Model file for the job. Use its own axes, mm. Face numbers are marked on the shaded views. A direction names the side the tool comes from. Coordinates: 2 decimals unless noted, no trailing zeros. Write each loop counter-clockwise with the first axis right and the second up, starting at its lowest first coordinate (ties: lowest second). Pieces come first, ordered by that corner, then holes. Notation, with made-up numbers: (65, 59.25) - (76, 59.25) arc R23 ccw to (76, 90.25) - close; hole circle Ø6 at (61.5, 86.25). An arc over 180 degrees is marked (long way). Put each result on its own line as item: value. Start each with the question number.
1. Which spindle directions (+Z, -Z, +X, -X, +Y, -Y) get a long thin tool onto all of the face, cutting with end or side? Do the marked faces 4, 5 and 6. Say none if no direction does.
2. Saw through at B-B, the plane y = 3.25. Write the cut outline in (x, z).
3. Saw through at A-A, the plane y = 0. Write the cut outline in (x, z).
4. Saw through at D-D, the plane x = 3. Write the cut outline in (y, z), plus the area to 3 significant figures.
5. Drop flat-ended pins along their axis: P1, Ø3, axis at y = 7.5, z = 3.5, coming from the -X side; P2, Ø3.5, axis at x = 3, y = 7.5, coming from the +Z side; P3, Ø4, axis at x = 1.5, y = 3, coming from the +Z side. Give the stop position or say it passes through.
6. Drill centre lines: L1, parallel to Z at x = -5.25, y = 6; L2, parallel to X at y = 11.75, z = 8.25; L3, parallel to Y at x = 0, z = 0.35. Where is each one in solid material? Low to high. Write a range as from..to.
7. Saw through at C-C, the plane z = 3.75. Write the cut outline in (x, y), plus the area to 3 significant figures.
8. Pull direction X, two halves, no side cores. Call the marked faces 1, 2 and 3: released by +X, released by -X, zero draft, split by the parting line, or undercut.
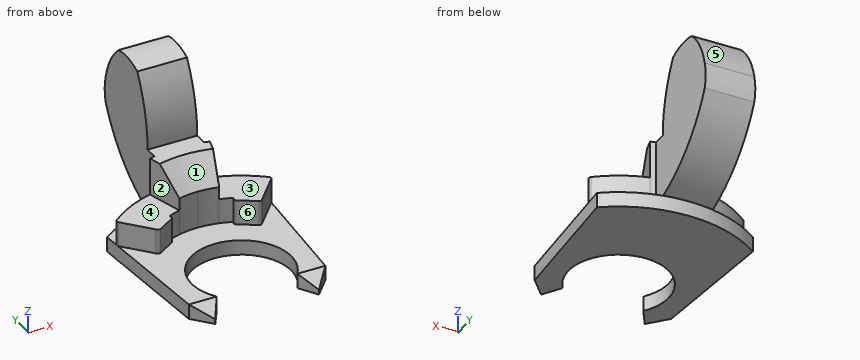
```python
from build123d import *

# Parameters (mm, degrees)
F1_DEPTH    = 1.2
F3_DEPTH    = 12.5
F5_DEPTH    = 2
F6_DEPTH    = 5
F7_T2_ANGLE = 119.2786087223
F8_DEPTH    = 5
F10_DEPTH   = 4
F11_DEPTH   = 5


# Not quite as in the source:
# - a fillet or chamfer that OpenCascade refuses, or shapes differently, is made with other operations: its cross-section is extruded or revolved along the edge and cut away or added
# - a feature names something its author has since deleted; it is built from what else it names


with BuildPart() as f1:
    # F0 (on Top) → F1 (new body)
    with BuildSketch(Plane.XY):
        with BuildLine():
            ThreePointArc((-3.25, -2.3318447633), (0, 4), (3.25, -2.3318447633))
            Line((3.25, -2.3318447633), (4.1771243445, -3.8318447633))
            Line((4.1771243445, -3.8318447633), (5.5, -2.3318447633))
            Line((5.5, -2.3318447633), (6.2861850371, 8.4103434936))
            ThreePointArc((6.2861850371, 8.4103434936), (0, 10.5), (-6.2861850371, 8.4103434936))
            Line((-6.2861850371, 8.4103434936), (-5.5, -2.3318447633))
            Line((-5.5, -2.3318447633), (-4.1771243445, -3.8318447633))
            Line((-4.1771243445, -3.8318447633), (-3.25, -2.3318447633))
        make_face()
    extrude(amount=F1_DEPTH)

    # F2 (on Right) → F3 (cut, symmetric)
    with BuildSketch(Plane.YZ):
        Polygon((-3.8318447633, 0.4), (-2.3318447633, 1.2), (-3.8318447633, 1.2), align=None)
    extrude(amount=F3_DEPTH, both=True, mode=Mode.SUBTRACT)

    # F4 (on face) → F5 (join)
    with BuildSketch(Plane.XY.offset(1.2)):
        with BuildLine():
            Line((0, 9.4893432962), (0, 9.5))
            ThreePointArc((0, 9.5), (-1.0056504861, 9.4466219941), (-2, 9.2870878105))
            ThreePointArc((-2, 9.2870878105), (-2.207287093, 9.2400153511), (-2.4134691055, 9.1883168686))
            Line((-2.4134691055, 9.1883168686), (-1.6054997382, 6.2986006851))
            ThreePointArc((-1.6054997382, 6.2986006851), (-0.809041268, 6.4494536378), (0, 6.5))
            Line((0, 6.5), (0, 9.4893432962))
        make_face()
        with BuildLine():
            Line((0, 10.3126084432), (0, 9.5))
            ThreePointArc((0, 9.5), (1.0056504861, 9.4466219941), (2, 9.2870878105))
            Line((2, 9.2870878105), (2, 10.3126084432))
            Line((2, 10.3126084432), (0, 10.3126084432))
        make_face()
        with BuildLine():
            ThreePointArc((2, 9.2870878105), (1.0056504861, 9.4466219941), (0, 9.5))
            Line((0, 9.5), (0, 9.4893432962))
            Line((0, 9.4893432962), (0, 6.5))
            ThreePointArc((0, 6.5), (0.809041268, 6.4494536378), (1.6054997382, 6.2986006851))
            Line((1.6054997382, 6.2986006851), (2.4134691055, 9.1883168686))
            ThreePointArc((2.4134691055, 9.1883168686), (2.207287093, 9.2400153511), (2, 9.2870878105))
        make_face()
        with BuildLine():
            ThreePointArc((-2, 9.2870878105), (-1.0056504861, 9.4466219941), (0, 9.5))
            Line((0, 9.5), (0, 10.3126084432))
            Line((0, 10.3126084432), (-2, 10.3126084432))
            Line((-2, 10.3126084432), (-2, 9.2870878105))
        make_face()
        with BuildLine():
            Line((-1.6054997382, 6.2986006851), (-2.4134691055, 9.1883168686))
            ThreePointArc((-2.4134691055, 9.1883168686), (-4.3834961594, 8.4282240965), (-6.1369591907, 7.2517399217))
            ThreePointArc((-6.1369591907, 7.2517399217), (-6.2072372931, 7.1135226449), (-6.1576144754, 6.9666192642))
            Line((-6.1576144754, 6.9666192642), (-4.3047045796, 4.8702688306))
            Line((-4.3047045796, 4.8702688306), (-4.2185888433, 4.7728389657))
            ThreePointArc((-4.2185888433, 4.7728389657), (-4.0971505607, 4.7073203992), (-3.9621862374, 4.7360357341))
            Line((-3.9621862374, 4.7360357341), (-2.5827247856, 5.6044208159))
            ThreePointArc((-2.5827247856, 5.6044208159), (-2.4942501859, 5.7293355978), (-2.5200172859, 5.8802246764))
            Line((-2.5200172859, 5.8802246764), (-2.5753119947, 5.968062343))
            ThreePointArc((-2.5753119947, 5.968062343), (-2.096928846, 6.152470188), (-1.6054997382, 6.2986006851))
        make_face()
        with BuildLine():
            ThreePointArc((6.1369591907, 7.2517399217), (4.3834961594, 8.4282240965), (2.4134691055, 9.1883168686))
            Line((2.4134691055, 9.1883168686), (1.6054997382, 6.2986006851))
            ThreePointArc((1.6054997382, 6.2986006851), (2.096928846, 6.152470188), (2.5753119947, 5.968062343))
            Line((2.5753119947, 5.968062343), (2.5200172859, 5.8802246764))
            ThreePointArc((2.5200172859, 5.8802246764), (2.4942501859, 5.7293355978), (2.5827247856, 5.6044208159))
            Line((2.5827247856, 5.6044208159), (3.9621862374, 4.7360357341))
            ThreePointArc((3.9621862374, 4.7360357341), (4.0971505607, 4.7073203992), (4.2185888433, 4.7728389657))
            Line((4.2185888433, 4.7728389657), (4.3047045796, 4.8702688306))
            Line((4.3047045796, 4.8702688306), (6.1576144754, 6.9666192642))
            ThreePointArc((6.1576144754, 6.9666192642), (6.2072372931, 7.1135226449), (6.1369591907, 7.2517399217))
        make_face()
    extrude(amount=F5_DEPTH)

    # F4 (on face) → F6 (join)
    with BuildSketch(Plane.XY.offset(1.2)):
        with BuildLine():
            ThreePointArc((2, 9.2870878105), (1.0056504861, 9.4466219941), (0, 9.5))
            Line((0, 9.5), (0, 9.4893432962))
            Line((0, 9.4893432962), (0, 6.5))
            ThreePointArc((0, 6.5), (0.809041268, 6.4494536378), (1.6054997382, 6.2986006851))
            Line((1.6054997382, 6.2986006851), (2.4134691055, 9.1883168686))
            ThreePointArc((2.4134691055, 9.1883168686), (2.207287093, 9.2400153511), (2, 9.2870878105))
        make_face()
        with BuildLine():
            Line((0, 9.4893432962), (0, 9.5))
            ThreePointArc((0, 9.5), (-1.0056504861, 9.4466219941), (-2, 9.2870878105))
            ThreePointArc((-2, 9.2870878105), (-2.207287093, 9.2400153511), (-2.4134691055, 9.1883168686))
            Line((-2.4134691055, 9.1883168686), (-1.6054997382, 6.2986006851))
            ThreePointArc((-1.6054997382, 6.2986006851), (-0.809041268, 6.4494536378), (0, 6.5))
            Line((0, 6.5), (0, 9.4893432962))
        make_face()
    extrude(amount=F6_DEPTH)

    # F7: chamfer of 2 on 1 edges, made by hand

    # F7_s1 → F7_t2 (revolve, cut)
    with BuildSketch(Plane(origin=(0, 0, 0), x_dir=(0, 0, 1), z_dir=(-0.5054419689, -0.8628606006, 0))):
        Polygon((6.2, 8.5), (4.2, 6.5), (6.2, 6.5), align=None)
    revolve(axis=Axis((0, 0, 6.2), (0, 0, -1)), revolution_arc=F7_T2_ANGLE, mode=Mode.SUBTRACT)

    # F4 (on face) → F8 (join, through all)
    with BuildSketch(Plane.XY.offset(1.2)):
        with BuildLine():
            Line((0, 10.3126084432), (0, 9.5))
            ThreePointArc((0, 9.5), (1.0056504861, 9.4466219941), (2, 9.2870878105))
            Line((2, 9.2870878105), (2, 10.307764064))
            ThreePointArc((2, 10.307764064), (1.9874359165, 10.3101939108), (1.974868881, 10.3126084432))
            Line((1.974868881, 10.3126084432), (0, 10.3126084432))
        make_face()
        with BuildLine():
            ThreePointArc((1.974868881, 10.3126084432), (1.9874359165, 10.3101939108), (2, 10.307764064))
            Line((2, 10.307764064), (2, 10.3126084432))
            Line((2, 10.3126084432), (1.974868881, 10.3126084432))
        make_face()
        with BuildLine():
            Line((-2, 10.3126084432), (-2, 10.307764064))
            ThreePointArc((-2, 10.307764064), (-1.9874359165, 10.3101939108), (-1.974868881, 10.3126084432))
            Line((-1.974868881, 10.3126084432), (-2, 10.3126084432))
        make_face()
        with BuildLine():
            ThreePointArc((-2, 9.2870878105), (-1.0056504861, 9.4466219941), (0, 9.5))
            Line((0, 9.5), (0, 10.3126084432))
            Line((0, 10.3126084432), (-1.974868881, 10.3126084432))
            ThreePointArc((-1.974868881, 10.3126084432), (-1.9874359165, 10.3101939108), (-2, 10.307764064))
            Line((-2, 10.307764064), (-2, 9.2870878105))
        make_face()
    extrude(amount=F8_DEPTH)

    # F9 (on face) → F10 (join)
    with BuildSketch(Plane(origin=(-2, 0, 0), x_dir=(0, -1, 0), z_dir=(-1, 0, 0))):
        with BuildLine():
            Line((-10.4906475171, 1.2), (-10.3126084432, 1.2))
            Line((-10.3126084432, 1.2), (-10.3126084432, 6.2))
            ThreePointArc((-10.3126084432, 6.2), (-10.7033019047, 9.142871965), (-11.848315427, 11.8818646297))
            ThreePointArc((-11.848315427, 11.8818646297), (-13.2228522743, 12.2616673302), (-14.6442650052, 12.1468305588))
            ThreePointArc((-14.6442650052, 12.1468305588), (-15.8696799602, 10.6519801079), (-16.5821556002, 8.8551500812))
            ThreePointArc((-16.5821556002, 8.8551500812), (-16.7217466821, 7.8095628414), (-16.5821556002, 6.7639756016))
            ThreePointArc((-16.5821556002, 6.7639756016), (-14.0870903715, 3.3790869985), (-10.4906475171, 1.2))
        make_face()
    extrude(amount=-F10_DEPTH)

    # F4 (on face) → F11 (join, through all)
    with BuildSketch(Plane.XY.offset(1.2)):
        with BuildLine():
            Line((0, 10.3126084432), (0, 9.5))
            ThreePointArc((0, 9.5), (1.0056504861, 9.4466219941), (2, 9.2870878105))
            Line((2, 9.2870878105), (2, 10.307764064))
            ThreePointArc((2, 10.307764064), (1.9874359165, 10.3101939108), (1.974868881, 10.3126084432))
            Line((1.974868881, 10.3126084432), (0, 10.3126084432))
        make_face()
        with BuildLine():
            ThreePointArc((-2, 9.2870878105), (-1.0056504861, 9.4466219941), (0, 9.5))
            Line((0, 9.5), (0, 10.3126084432))
            Line((0, 10.3126084432), (-1.974868881, 10.3126084432))
            ThreePointArc((-1.974868881, 10.3126084432), (-1.9874359165, 10.3101939108), (-2, 10.307764064))
            Line((-2, 10.307764064), (-2, 9.2870878105))
        make_face()
    extrude(amount=F11_DEPTH)


solid = f1.part
```
Final values:
1. face 4: +Z, -X, -Y
1. face 5: +Z, +X, -X, +Y
1. face 6: +Z, -Y
2. outline: (-5.91, 0) - (-2.33, 0) - (-2.33, 1.2) - (-5.91, 1.2) - close; (2.33, 0) - (5.91, 0) - (5.91, 1.2) - (2.33, 1.2) - close
3. outline: (-5.67, 0) - (-4, 0) - (-4, 1.2) - (-5.67, 1.2) - close; (4, 0) - (5.67, 0) - (5.67, 1.2) - (4, 1.2) - close
4. outline: (2.65, 0) - (10.06, 0) - (10.06, 1.2) - (9.01, 1.2) - (9.01, 3.2) - (5.34, 3.2) - (5.34, 1.2) - (2.65, 1.2) - close
4. area: 16.2 mm²
5. P1: stops at x = -6.21
5. P2: stops at z = 6.2
5. P3: stops at z = 1.2
6. L1: z = 0..3.2
6. L2: x = -2..2
6. L3: y = 4..10.5
7. outline: (-2.41, 9.19) - (-1.61, 6.3) arc R6.5 cw to (1.61, 6.3) - (2.41, 9.19) arc R9.5 ccw to (2, 9.29) - (2, 14.47) - (-2, 14.47) - (-2, 9.29) arc R9.5 ccw to start
7. area: 32.4 mm²
8. face 1: undercut
8. face 2: released by -X
8. face 3: zero draft
